```python
from build123d import *

# Parameters (mm, degrees)
SKETCH1_W             = 60
SKETCH1_H             = 60
BOSS_EXTRUDE1_DEPTH   = 22
SKETCH2_R             = 3
CUT_EXTRUDE1_DEPTH    = 23
CHAMFER1_SIZE         = 3
FILLET1_R             = 8
M4X0_7_TAPPED_HOLE1_D = 3.3


with BuildPart() as part:
    # Sketch1 → Boss-Extrude1 (new body)
    with BuildSketch(Plane.XY):
        Rectangle(SKETCH1_W, SKETCH1_H)
    extrude(amount=BOSS_EXTRUDE1_DEPTH)

    # Sketch2 → Cut-Extrude1 (cut, through all)
    with BuildSketch(Plane(origin=(0, 0, 0), x_dir=(-1, 0, 0), z_dir=(0, 0, -1))):
        Circle(SKETCH2_R)
    extrude(amount=-CUT_EXTRUDE1_DEPTH, mode=Mode.SUBTRACT)

    # Chamfer1
    chamfer1_edges = [part.edges().sort_by_distance(p)[0] for p in [
        (3, 0, 0),
    ]]
    chamfer(chamfer1_edges, length=CHAMFER1_SIZE)

    # Fillet1
    fillet1_edges = [part.edges().sort_by_distance(p)[0] for p in [
        (30, -30, 11),
        (-30, -30, 11),
        (-30, 30, 11),
        (30, 30, 11),
    ]]
    fillet(fillet1_edges, radius=FILLET1_R)

    # M4x0.7 Tapped Hole1 (through all)
    with Locations(Plane(origin=(0, 0, 0), x_dir=(-1, 0, 0), z_dir=(0, 0, -1))):
        with Locations((-22, 22), (22, 22), (22, -22), (-22, -22)):
            Hole(M4X0_7_TAPPED_HOLE1_D / 2)


solid = part.part
```
Design review of the part built by this model. Coordinates are the model's own, in mm. Coordinates: 2 decimals unless noted, no trailing zeros. Order: outer loops, then holes, each group sorted by start corner. A loop starts at its lowest first (then second) coordinate and runs counter-clockwise, first axis right, second up. Notation, with made-up numbers: M 84,59.5 L 93,59.5 A17 cw 93,64.5 Z; hole C 63.25,44.5 d6. An arc over 180 degrees is marked long. Answer as a JSON object with one key per item and string values. Group by question number.
1) Wall thickness on L1, parallel to Y at x = 22, z = 9.5; L2, parallel to Y at x = 0, z = 14.5; L3, parallel to X at y = 0, z = 2: over which ranges is each line inside the solid? List them lowest first.
2) Mouldability with a two-part tool opening along Y and no side actions: class faces 1 (the flat face through (-7, 0, 0)), 2 (the flat face through (0, -30, 11)), 3 (the cylindrical face through (27.594, 27.719, 11.154)), 4 (the conical face through (0.682, -3.071, 2.854)) as pulls with the +Y half, pulls with the -Y half, needs draft (parallel to the pull), parting line crosses it, or undercut.
3) Add section D-D, the plane x = 25.5. Write out the cut boundary in (y, z).
4) Add section C-C, the plane z = 11.25. Write out the cut boundary in (x, y), then the cut area to 3 significant figures.
5) Add section A-A, the plane x = 0. Write out the cut boundary in (y, z), then the cut area to 3 significant figures.
Computed values:
{
 "1": {"L1": "y = -30 to -23.65, -20.35 to 20.35, 23.65 to 30", "L2": "y = -30 to -3, 3 to 30", "L3": "x = -30 to -4, 4 to 30"},
 "2": {"face 1": "needs draft", "face 2": "pulls with the -Y half", "face 3": "pulls with the +Y half", "face 4": "undercut"},
 "3": {"outline": "M -29.19,0 L 29.19,0 L 29.19,22 L -29.19,22 Z"},
 "4": {"outline": "M -30,-22 A8 ccw -22,-30 L 22,-30 A8 ccw 30,-22 L 30,22 A8 ccw 22,30 L -22,30 A8 ccw -30,22 Z; hole C -22,-22 d3.3; hole C -22,22 d3.3; hole C 0,0 d6; hole C 22,-22 d3.3; hole C 22,22 d3.3", "area": "3,480 mm^2"},
 "5": {"outline": "M -30,0 L -6,0 L -3,3 L -3,22 L -30,22 Z; M 3,3 L 6,0 L 30,0 L 30,22 L 3,22 Z", "area": "1,180 mm^2"}
}
